```python
from build123d import *

# Parameters (mm, degrees)
SKETCH1_W           = 40
SKETCH1_H           = 40
SKETCH1_R           = 3.1
BOSS_EXTRUDE1_DEPTH = 3
BOSS_EXTRUDE2_DEPTH = 40


with BuildPart() as part:
    # Sketch1 → Boss-Extrude1 (new body)
    with BuildSketch(Plane(origin=(0, 0, 0), x_dir=(1, 0, 0), z_dir=(0, 1, 0))):
        Rectangle(SKETCH1_W, SKETCH1_H)
        with Locations(Location((0, 0, 0), (0, 0, 270))):
            Circle(SKETCH1_R, mode=Mode.SUBTRACT)
    extrude(amount=BOSS_EXTRUDE1_DEPTH)

    # Sketch6 → Boss-Extrude2 (add)
    with BuildSketch(Plane(origin=(0, 0, -20), x_dir=(-1, 0, 0), z_dir=(0, 0, -1))):
        Polygon((-109.619318504, 39.815596494), (-20, 0), (-20, 3), (-110.058959884, 42.815596494), align=None)
    extrude(amount=-BOSS_EXTRUDE2_DEPTH)


solid = part.part
```
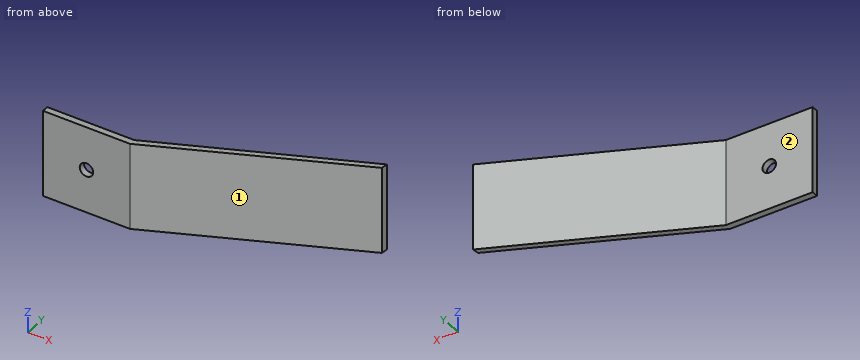
Source: CAD feature listing. Evaluate the final solid. Frame: model axes, mm. Face numbers are marked on the shaded views. A direction names the side the tool comes from. Coordinates: 2 decimals unless noted, no trailing zeros. Write each loop counter-clockwise with the first axis right and the second up, starting at its lowest first coordinate (ties: lowest second). Pieces come first, ordered by that corner, then holes. Notation, with made-up numbers: (62.25, 61.5) - (83.25, 61.5) arc R20 cw to (83.25, 87.5) - close; hole circle Ø6 at (87.5, 72). An arc over 180 degrees is marked (long way). Answer as a JSON object with one key per item and string values.
Q1. Section query A-A, the plane z = 0. Output: boundary loops of the cut face in (x, y).
Ans:
{"outline": "(-20, 0) - (-3.1, 0) - (-3.1, 3) - (-20, 3) - close; (3.1, 0) - (20, 0) - (109.62, 39.82) - (110.06, 42.82) - (20, 3) - (3.1, 3) - close"}
Q2. Material intervals for line 1 (Y direction, x = 2, z = -9.5); line 2 (X direction, y = 1.05, z = 0); line 3 (X direction, y = 2.35, z = 0), sorted ascending. Write a range as [from, to].
Ans:
{"line 1": "y = [0, 3]", "line 2": "x = [-20, -3.1], [3.1, 22.36]", "line 3": "x = [-20, -3.1], [3.1, 25.29]"}
Q3. Section query C-C, the plane z = 17. Output: boundary loops of the cut face in (x, y).
Ans:
{"outline": "(-20, 0) - (20, 0) - (109.62, 39.82) - (110.06, 42.82) - (20, 3) - (-20, 3) - close"}
Q4. First-contact query: pin 1 Ø8 at (y, z) = (19.5, -13.5) entering from -X; pin 2 Ø6 at (y, z) = (6.5, -10) entering from +X; pin 3 Ø10 at (x, z) = (24.5, -4) entering from -Y; pin 4 Ø1 at (y, z) = (29, -5.5) entering from +X. Flat tips, straight axial feed; report the tip coordinate or a pass-through.
Ans:
{"pin 1": "stops at x = 48.27", "pin 2": "stops at x = 41.38", "pin 3": "stops at y = 0", "pin 4": "stops at x = 86.4"}
Q5. Set-up query: the marked faces 1 and 2. Return all of +Z, -Z, +X, -X, +Y, -Y with unobstructed straight access to the full face (end or side cutting, diameter ignored); none if empty.
Ans:
{"face 1": "+Z, -Z, +X, -Y", "face 2": "+Z, -Z, -X, +Y"}
Q6. Section query B-B, the plane x = 0. Output: boundary loops of the cut face in (y, z).
Ans:
{"outline": "(0, -20) - (3, -20) - (3, -3.1) - (0, -3.1) - close; (0, 3.1) - (3, 3.1) - (3, 20) - (0, 20) - close"}
Q7. Section query D-D, the plane x = 77.5. Output: boundary loops of the cut face in (y, z).
Ans:
{"outline": "(25.55, -20) - (28.42, -20) - (28.42, 20) - (25.55, 20) - close"}
